The listing builds one solid part. Answer for the finished solid, in the listing's coordinates (mm). A direction names the side the tool comes from. Coordinates: 2 decimals unless noted, no trailing zeros. Write each loop counter-clockwise with the first axis right and the second up, starting at its lowest first coordinate (ties: lowest second). Pieces come first, ordered by that corner, then holes.
from build123d import *

# Parameters (mm, degrees)
F0_W     = 9.525
F0_H     = 23.8125
F1_DEPTH = 7.9375
F2_R     = 3.96874
F3_W     = 23.8125
F3_H     = 3.96875
F4_DEPTH = 15.875
F5_W     = 1.6891
F5_H     = 1.56845
F5_H_2   = 1.6891
F5_W_2   = 1.56845
F5_R     = 2.54
F6_DEPTH = 31.75


# Not quite as in the source:
# - a fillet or chamfer is up to 0.001 mm smaller than in the source, because OpenCascade refuses the exact size


with BuildPart() as f1:
    # F0 (on Top) → F1 (new body)
    with BuildSketch(Plane.XY):
        with Locations((-4.7625, -11.90625)):
            Rectangle(F0_W, F0_H)
        Polygon((-9.525, -23.8125), (-9.525, 0), (-9.525, 3.96875), (-111.125, 3.96875), (-111.125, -27.78125), (-9.525, -27.78125), align=None)
    extrude(amount=F1_DEPTH)

    # F2 (radius 3.96875 in the source; OpenCascade refuses exactly that, so slightly less here)
    f2_edges = [f1.edges().sort_by_distance(p)[0] for p in [
        (-9.525, -25.796875, 7.9375),
        (-9.525, -25.796875, 0),
        (0, -11.90625, 7.9375),
        (0, -11.90625, 0),
        (-9.525, 1.984375, 7.9375),
        (-9.525, 1.984375, 0),
    ]]
    fillet(f2_edges, radius=F2_R)

    # F3 (on face) → F4 (join)
    with BuildSketch(Plane.XY.offset(7.9375)):
        with Locations((-67.46875, -21.828125)):
            Rectangle(F3_W, F3_H)
        with Locations((-67.46875, -1.984375)):
            Rectangle(F3_W, F3_H)
    extrude(amount=F4_DEPTH)

    # F5 (on face) → F6 (cut, through all)
    with BuildSketch(Plane.XZ.offset(27.78125)):
        with BuildLine():
            Line((-55.5625, 23.8125), (-59.53125, 23.8125))
            ThreePointArc((-59.53125, 23.8125), (-56.7249199622, 22.6500800378), (-55.5625, 19.84375))
            Line((-55.5625, 19.84375), (-55.5625, 23.8125))
        make_face()
        with BuildLine():
            Line((-59.53125, 23.8125), (-79.375, 23.8125))
            Line((-79.375, 23.8125), (-79.375, 7.9375))
            Line((-79.375, 7.9375), (-62.126542618, 22.8463210299))
            ThreePointArc((-62.126542618, 22.8463210299), (-60.915902084, 23.5631202651), (-59.53125, 23.8125))
        make_face()
        with Locations((-59.53125, 18.214975)):
            Rectangle(F5_W, F5_H)
        with Locations((-59.53125, 19.84375)):
            Rectangle(F5_W, F5_H_2)
        with Locations((-57.902475, 19.84375)):
            Rectangle(F5_W_2, F5_H_2)
        with Locations((-61.160025, 19.84375)):
            Rectangle(F5_W_2, F5_H_2)
        with Locations((-59.53125, 21.472525)):
            Rectangle(F5_W, F5_H)
        with Locations((-3.96875, 3.96875)):
            Circle(F5_R)
    extrude(amount=-F6_DEPTH, mode=Mode.SUBTRACT)


solid = f1.part
Q1. The part is cut by section C-C, the plane x = -44.5. Write down the section's boundary in (y, z).
Answers below:
outline: (-27.78, 0) - (3.97, 0) - (3.97, 7.94) - (-27.78, 7.94) - close
Q2. Which of the six approach directions +Z, -Z, +X, -X, +Y, -Y give full straight-line access (tool end or side, diameter ignored) to faces 1 (the face through (-65, -3.969, 14)), 2 (the face through (-10.657, 2.012, 6.744)), 3 (the face through (-58, -12, 0)), 4 (the face through (-10.66, 2.01, 1.19)), 5 (the face through (-55.562, -2, 14))?
Answers below:
face 1: +Z, +X, -X
face 2: +Z, +X, +Y
face 3: -Z, +X, -X, +Y, -Y
face 4: -Z, +X, +Y
face 5: +Z, +X, +Y, -Y
Q3. The part is cut by section D-D, the plane z = 11. Write down the section's boundary in (x, y).
Answers below:
outline: (-75.83, -23.81) - (-55.56, -23.81) - (-55.56, -19.84) - (-75.83, -19.84) - close; (-75.83, -3.97) - (-55.56, -3.97) - (-55.56, 0) - (-75.83, 0) - close
Q4. Given pin 1 (12 mm diameter, centred on y = -22, z = 16.5, fed in from -X); pin 2 (1.4 mm diameter, centred on y = -21.5, z = 20, fed in from -X); pin 3 (4 mm diameter, centred on x = -5, z = 3.5, fed in from +Y); pin 4 (12 mm diameter, centred on x = -12.5, z = 15.5, fed in from +Y), each flat-ended and moving along its own axis, determine where each tip first touches the part or whether it passes through.
Answers below:
pin 1: stops at x = -76.41
pin 2: stops at x = -66.23
pin 3: stops at y = 0
pin 4: passes through
Q5. Find the intervals of material crossed by probe 1 along Y at (x, z) = (-58, 11.25); probe 2 along Z at (x, y) = (-25, -9.5); probe 3 along X at (y, z) = (-2.5, 4.75) (3 decimals), in increasing order.
Answers below:
probe 1: y = -23.81 to -19.84, -3.97 to 0
probe 2: z = 0 to 7.94
probe 3: x = -111.125 to -6.386, -1.552 to -0.078
Q6. Determine the mould class of faces 6 (the face through (-7, -23.812, 4)), 7 (the face through (-10.66, -25.77, 1.19)), 8 (the face through (-58, -12, 7.938)) for opening direction Y: released by +Y, released by -Y, zero draft, split by the parting line, or undercut.
Answers below:
face 6: released by -Y
face 7: zero draft
face 8: undercut
Q7. The part is cut by section B-B, the plane z = 5.5. Write down the section's boundary in (x, y) (1 decimal).
Answers below:
outline: (-111.1, -27.8) - (-9.8, -27.8) - (-9.8, -23.8) - (-6, -23.8) - (-6, 0) - (-9.8, 0) - (-9.8, 4) - (-111.1, 4) - close; (-1.9, -23.8) - (-0.3, -23.8) - (-0.3, 0) - (-1.9, 0) - close
